Part print with two shaded views. Sizes in mm from the minimum x, y, z corner. Coordinates: 2 decimals unless noted, no trailing zeros. Loops run counter-clockwise (first coordinate to the right, second up) from the corner with the lowest first, then second, coordinate; pieces in that order, holes last.
(1) Slice it at B-B (y = 49.5). Give the cut face in (x, z), and give its area (3 significant figures).
(2) Slice it at A-A (z = 399). Give the cut face in (x, y).
(3) Slice it at D-D (x = 619.5). Give the cut face in (y, z).
(4) Flat gauge pin, fed straight in: P1, Ø23, axis at y = 452, z = 748, coming from the +X side. Where does the tip first touch, or does it go through?
(5) Slice it at C-C (x = 516). Give the cut face in (y, z), and give its area (3 significant figures).
(6) Wall check: L1, parallel to Z at x = 66, y = 716.5; L2, parallel to X at y = 479.5, z = 564; L3, parallel to Y at x = 48, z = 967. Give the ranges that are in metal, low to high.
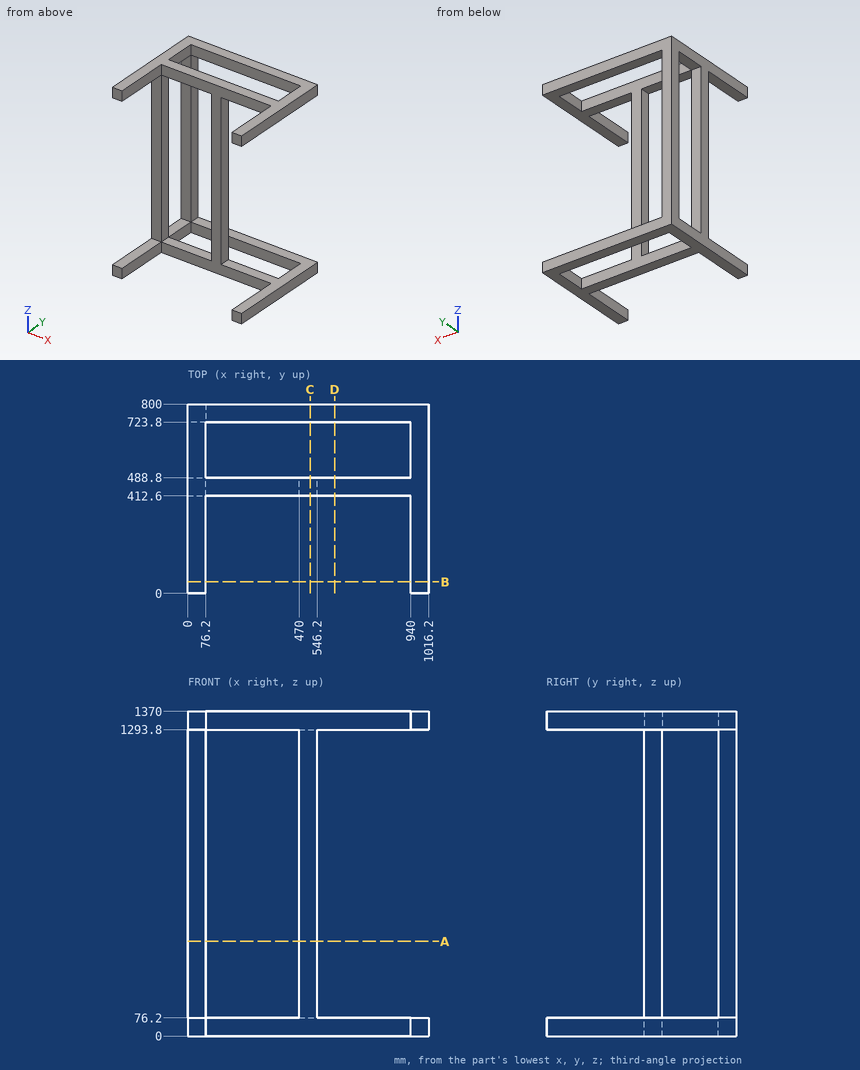
Response values:
1. outline: (0, 0) - (76.2, 0) - (76.2, 76.2) - (0, 76.2) - close; (0, 1293.8) - (76.2, 1293.8) - (76.2, 1370) - (0, 1370) - close; (940, 0) - (1016.2, 0) - (1016.2, 76.2) - (940, 76.2) - close; (940, 1293.8) - (1016.2, 1293.8) - (1016.2, 1370) - (940, 1370) - close
1. area: 23,200 mm2
2. outline: (0, 412.6) - (76.2, 412.6) - (76.2, 488.8) - (0, 488.8) - close; (0, 723.8) - (76.2, 723.8) - (76.2, 800) - (0, 800) - close; (470, 412.6) - (546.2, 412.6) - (546.2, 488.8) - (470, 488.8) - close
3. outline: (412.6, 0) - (488.8, 0) - (488.8, 76.2) - (412.6, 76.2) - close; (412.6, 1293.8) - (488.8, 1293.8) - (488.8, 1370) - (412.6, 1370) - close; (723.8, 0) - (800, 0) - (800, 76.2) - (723.8, 76.2) - close; (723.8, 1293.8) - (800, 1293.8) - (800, 1370) - (723.8, 1370) - close
4. P1: stops at x = 546.2
5. outline: (412.6, 0) - (488.8, 0) - (488.8, 1370) - (412.6, 1370) - close; (723.8, 0) - (800, 0) - (800, 76.2) - (723.8, 76.2) - close; (723.8, 1293.8) - (800, 1293.8) - (800, 1370) - (723.8, 1370) - close
5. area: 116,000 mm2
6. L1: z = 0 to 76.2, 1293.8 to 1370
6. L2: x = 0 to 76.2, 470 to 546.2
6. L3: y = 412.6 to 488.8, 723.8 to 800
